Autodesk Inventor part; units mm, degrees
ref_plane "YZ Plane" through (0, 0, 0) normal (1, 0, 0) x (0, 1, 0)
ref_plane "XZ Plane" through (0, 0, 0) normal (0, 1, 0) x (-1, 0, 0)
ref_plane "XY Plane" through (0, 0, 0) normal (0, 0, 1) x (1, 0, 0)
ref_plane "Work Plane1" through (1143.7783, 851.9673, -406.3915) normal (0, 0, -1) x (-0.8080578, -0.5891032, 0)
sketch "Sketch1" plane through (1143.7783, 851.9673, -406.3915) normal (0, 0, -1) x (-0.8080578, -0.5891032, 0)
  line L0 (1269.8194, 209.303) -> (1593.8019, 73.5805)
  line L1 (1593.8019, 73.5805) -> (1269.8194, -281.049)
  line L2 (1259.4205, 173.4665) -> (1567.246, 44.5125)
  line L3 (1511.4503, 67.8864) -> (1259.4205, -207.9841)
  line L4 (1259.4205, 213.6593) -> (1259.4205, 173.4665)
  line L5 (1259.4205, -207.9841) -> (1269.8194, -281.049)
  point P0 (1426.1356, -14.6355)
extrude "Extrusion1" add sketch "Sketch1" against normal blind 25.4
ref_plane "Work Plane3" through (1143.7783, 851.9673, -406.3915) normal (0, 0, -1) x (-0.8080578, -0.5891032, 0)
sketch "Sketch3" plane through (1143.7783, 851.9673, -406.3915) normal (0, 0, -1) x (-0.8080578, -0.5891032, 0)
  line L0 (1264.3348, 241.5423) -> (1610.7303, 93.3818)
  line L1 (1511.4503, 67.8864) -> (1567.246, 44.5125)
  line L2 (1610.7303, 93.3818) -> (1567.246, 44.5125)
  line L3 (1567.246, 44.5125) -> (1264.3348, 174.0739)
  line L4 (1264.3348, 174.0739) -> (1264.3348, 241.5423)
  point P0 (1426.1356, -14.6355)
extrude "Extrusion3" add sketch "Sketch3" against normal blind 25.4
ref_plane "Work Plane4" through (1129.2131, 527.0149, 254.0085) normal (0, 0, 1) x (0.8080578, 0.5891032, 0)
sketch "Sketch4" plane through (1129.2131, 527.0149, 254.0085) normal (0, 0, 1) x (0.8080578, 0.5891032, 0)
  line L0 (-1061.1348, 428.0739) -> (-1061.1348, 495.5423)
  line L1 (-1061.1348, 495.5423) -> (-1407.5303, 347.3818)
  line L2 (-1061.1348, 495.5423) -> (-1407.5303, 347.3818)
  line L3 (-1364.046, 298.5125) -> (-1066.6194, -27.049)
  line L4 (-1407.5303, 347.3818) -> (-1066.6194, -27.049)
  line L5 (-1066.6194, -27.049) -> (-1066.6194, 56.4973)
  line L6 (-1308.2503, 321.8864) -> (-1364.046, 298.5125)
  line L7 (-1066.6194, 56.4973) -> (-1308.2503, 321.8864)
  line L8 (-1364.046, 298.5125) -> (-1061.1348, 428.0739)
  line L9 (-1308.2503, 321.8864) -> (-1061.1348, 428.0739)
  line L10 (-1061.1348, 428.0739) -> (-1061.1348, 495.5423)
  line L11 (-1407.5303, 347.3818) -> (-1364.046, 298.5125)
  line L12 (-1407.5303, 347.3818) -> (-1343.0061, 374.9801)
  line L13 (-1308.2503, 321.8864) -> (-1364.046, 298.5125)
  point P0 (-1222.9356, 239.3645)
  point P1 (-1364.046, 298.5125)
  point P2 (-1293.9365, 306.2186)
extrude "Extrusion4" add sketch "Sketch4" against normal blind 25.4 contours L8 L4 L1 L0 | L9 L6 L4 L8 | L7 L5 L4 L6
sketch "Sketch5" plane through (1143.7783, 851.9673, -380.9915) normal (0, 0, 1) x (0.8080578, 0.5891032, 0)
  line L0 (-1567.246, 44.5125) -> (-1264.3348, 174.0739)
  line L1 (-1514.0603, 67.2611) -> (-1559.35, 115.3583)
  line L2 (-1264.3348, 241.5423) -> (-1610.7303, 93.3818)
  line L3 (-1610.7303, 93.3818) -> (-1559.35, 38.8164)
  line L4 (-1559.35, 38.8164) -> (-1521.1481, 74.7883)
  point P0 (-1426.1356, -14.6355)
  point P1 (-1264.3348, 174.0739)
  point P2 (-1584.1346, -28.1729)
extrude "Extrusion5" add sketch "Sketch5" along normal blind 635 contours L3 L2 L1 L4 L0 | L0 L4 L3
properties part number "RearCrumple"
Input: part model. Units: mm. Frame: model coordinates. A direction names the side the tool comes from. Coordinates: 2 decimals unless noted, no trailing zeros. Loops run counter-clockwise (first coordinate to the right, second up) from the corner with the lowest first, then second, coordinate; pieces in that order, holes last.
(1) Set-up query: faces 1 (the face through (-176.481, -28.276, -80.459)), 2 (the face through (-134.362, -9.86, -80.459)), 3 (the face through (-156.457, 21.354, -80.459)), 4 (the face through (-132.99, -9.09, -393.87)). Return all of +Z, -Z, +X, -X, +Y, -Y with unobstructed straight access to the full face (end or side cutting, diameter ignored); none if empty.
(2) Pull-direction query (Y, two-part tool) for faces 5 (the face through (265.695, -90.152, -393.869)), 6 (the face through (74, -59, -380.992)), 7 (the face through (-181.28, -28.3, -393.87)), 8 (the face through (62.97, -20.28, -393.87)); classes: released by +Y, released by -Y, zero draft, split by the parting line, or undercut.
(3) Section B-B on y = 87.5. Return the cut outline in (x, z).
(4) Section C-C on y = 271. Return the cut outline in (x, z).
(5) First-contact query: pin 1 Ø15.5 at (x, y) = (-184, -28.5) entering from +Z; pin 2 Ø2 at (y, z) = (-38, -340) entering from +X (1 decimal). Flat tips, straight axial feed; report the tip coordinate or a pass-through.
(6) Section D-D on z = -127. Return the cut outline in (x, y).
(7) Section A-A on x = 2. Return the cut outline in (y, z).
(8) Material intervals for probe 1 along Z at (x, y) = (-63.5, 179.5); probe 2 along X at (y, z) = (9, 93.5); probe 3 along X at (y, z) = (12, -29.5), sorted ascending.
Data:
1. face 1: -X, -Y
1. face 2: +X, -Y
1. face 3: +X, +Y
1. face 4: none
2. face 5: released by +Y
2. face 6: zero draft
2. face 7: released by -Y
2. face 8: undercut
3. outline: (-147.97, -406.39) - (-75.79, -406.39) - (-75.79, -380.99) - (-147.97, -380.99) - close; (-147.97, 228.61) - (-75.43, 228.61) - (-75.43, 254.01) - (-147.97, 254.01) - close
4. outline: (-38.81, -406.39) - (2.67, -406.39) - (2.67, -380.99) - (-38.81, -380.99) - close; (-38.81, 228.61) - (2.67, 228.61) - (2.67, 254.01) - (-38.81, 254.01) - close
5. pin 1: stops at z = 254.01
5. pin 2: passes through
6. outline: (-212.8, -21.46) - (-139.13, -35.28) - (-129.46, 16.29) - (-184.22, 26.57) - close
7. outline: (-66.01, -406.39) - (-7.88, -406.39) - (-7.88, -380.99) - (-66.01, -380.99) - close; (-65.51, 228.61) - (-8.09, 228.61) - (-8.09, 254.01) - (-65.51, 254.01) - close; (218.15, 228.61) - (271.91, 228.61) - (271.91, 254.01) - (218.15, 254.01) - close; (218.26, -406.39) - (271.91, -406.39) - (271.91, -380.99) - (218.26, -380.99) - close
8. probe 1: z = -406.39 to -380.99, 228.61 to 254.01
8. probe 2: x = -194.67 to -130.82
8. probe 3: x = -192.89 to -130.26
